Autodesk Inventor part; units mm, degrees
ref_plane "YZ Plane" through (0, 0, 0) normal (1, 0, 0) x (0, 1, 0)
ref_plane "XZ Plane" through (0, 0, 0) normal (0, 1, 0) x (-1, 0, 0)
ref_plane "XY Plane" through (0, 0, 0) normal (0, 0, 1) x (1, 0, 0)
sketch "Sketch1" plane through (0, 0, 0) normal (0, 1, 0) x (-1, 0, 0)
  line L0 (10, -18.5) -> (-10, -18.5)
  line L1 (-10, -18.5) -> (-10, 18.5)
  line L2 (-10, 18.5) -> (10, 18.5)
  line L3 (10, 18.5) -> (10, -18.5)
  point P0 (0, 0)
  dimension "d0" = 20
  dimension "d1" = 37
  dimension "d2" = 18.5
  dimension "d3" = 10
extrude "Plate1" add sketch "Sketch1" along normal blind 1.5
sketch "Sketch2" plane through (-10, 0, -20) normal (0, 0, 1) x (1, 0, 0)
  line L0 (20, 0) -> (0, 0)
  line L1 (0, 0) -> (0, 51.6)
  line L2 (0, 51.6) -> (20, 51.6)
  line L3 (20, 51.6) -> (20, 0)
edge flange "Flange1" height 51.6 angle 90 thickness 1.5 bend radius 0.31 thickness toward (0, 0, 1) relief tear relief width 1.5 relief depth 0.75 edges at (0, 1.5, -18.5) wall of the first edge with corners at (10, 0, -20) (-10, 0, -20) (-10, 51.6, -20) (10, 51.6, -20)
bend "Bend1"
corner "Corner1"
sketch "Sketch3" plane through (10, 0, 20) normal (0, 0, -1) x (-1, 0, 0)
  line L0 (20, 0) -> (0, 0)
  line L1 (0, 0) -> (0, 51.6)
  line L2 (0, 51.6) -> (20, 51.6)
  line L3 (20, 51.6) -> (20, 0)
edge flange "Flange2" height 51.6 angle 90 thickness 1.5 bend radius 0.31 thickness toward (0, 0, -1) relief tear relief width 1.5 relief depth 0.75 edges at (0, 1.5, 18.5) wall of the first edge with corners at (-10, 0, 20) (10, 0, 20) (10, 51.6, 20) (-10, 51.6, 20)
bend "Bend2"
corner "Corner2"
sketch "Sketch4" plane through (-10, 51.6, 20) normal (0, 0, 1) x (1, 0, 0)
  circle A0 centre (10, -10) radius 10
  line L0 (0, 0) -> (20, 0)
  line L1 (0, 0) -> (20, 0)
  line L2 (20, 0) -> (20, -10)
  line L3 (20, -10) -> (0, -10)
  line L4 (0, -10) -> (0, 0)
  line L5 (0, -49.79) -> (0, 0)
  point P0 (10, -51.6)
  point P1 (10, 0)
  dimension "d26" = 20
  dimension "d25" = 10
  dimension "d27" = 10
  dimension "d28" = 10
extrude "Extrusion1" cut sketch "Sketch4" against normal blind 10 contours L4 L0 A0 | A0 L0 L2
sketch "Sketch5" plane through (10, 51.6, -20) normal (0, 0, -1) x (-1, 0, 0)
  arc A0 (20, -10) -> (0, -10) centre (10, -10) ccw
  point P0 (10, -51.6)
hole "Hole1" at (0, 41.6, -20) direction (0, 0, 1) diameter 12.8 depth 1.5
sketch "Sketch6" plane through (10, 51.6, -20) normal (0, 0, -1) x (-1, 0, 0)
  line L0 (0, 0) -> (20, 0)
  circle A0 centre (10, -10) radius 6.4
  line L1 (-4, 0) -> (24, 0)
  line L2 (24, 0) -> (24, -10)
  line L3 (24, -10) -> (-4, -10)
  line L4 (-4, -10) -> (-4, 0)
  line L5 (0, -49.79) -> (0, 0)
  line L6 (0, -49.79) -> (20, -49.79)
  point P0 (10, -51.6)
  dimension "d38" = 28
  dimension "d39" = 10
  dimension "d40" = 4
  dimension "d41" = 49.79
extrude "Extrusion2" cut sketch "Sketch6" against normal blind 10 contours L5 L3 L4 L1 | L0 L1 L2 L3 A0 L5 | A0 L3 picked at (9.2435, -8.0053)
sketch "Sketch7" plane through (-10, 1.81, -18.5) normal (0, 0, 1) x (1, 0, 0)
  circle A0 centre (10, 12.37) radius 0.7835
  circle A1 centre (17, 19.67) radius 0.7835
  line L0 (16.4, 39.79) -> (20, 39.79)
  line L1 (20, 0) -> (20, 39.79)
  line L2 (20, 0) -> (0, 0)
  line L3 (0, 39.79) -> (0, 0)
  line L4 (0, 39.79) -> (3.6, 39.79)
  arc A2 (3.6, 39.79) -> (16.4, 39.79) centre (10, 39.79) ccw
  circle A3 centre (3, 19.67) radius 0.7835
  circle A4 centre (2, 32.89) radius 0.7835
  circle A5 centre (18, 32.89) radius 0.7835
  point P0 (10, -1.81)
hole "Hole2" at (0, 14.18, -18.5) at (-7, 21.48, -18.5) at (-8, 34.7, -18.5) at (8, 34.7, -18.5) at (7, 21.48, -18.5) direction (0, 0, -1) diameter 2.1 depth 1.5
fillet "Fillet1" radius 1 2 edges at (-10, 41.6, -19.25) (10, 41.6, -19.25)
sketch "Sketch8" plane through (-10, 1.81, 20) normal (0, 0, 1) x (1, 0, 0)
  arc A0 (20, 39.79) -> (0, 39.79) centre (10, 39.79) ccw
  point P0 (10, -1.81)
hole "Hole3" at (0, 41.6, 20) direction (0, 0, -1) diameter 3 depth 1.5
sketch "Sketch9" plane through (0, 0, 0) normal (0, -1, 0) x (1, 0, 0)
  line L0 (10.07, -24.6) -> (10.07, 7.5)
  line L1 (10, 20) -> (-10, 20)
  line L2 (10, 18.19) -> (10, -18.19)
  point P0 (0, 0)
  point P1 (8, 9.5)
  point P2 (8, -6.5)
  point P3 (-8, 9.5)
  point P4 (-8, -6.5)
  dimension "d59" = 2
  dimension "d60" = 10.5
  dimension "d63" = 16
  dimension "d66" = 16
hole "Hole4" at (8, 0, 9.5) at (8, 0, -6.5) at (-8, 0, 9.5) at (-8, 0, -6.5) direction (0, 1, 0) diameter 2.1 depth 1.5
equation "\"d36\" = Thickness"
equation "\"d49\" = Thickness"
equation "\"d57\" = Thickness"
equation "\"d74\" = Thickness"
equation "\"d4\" = Thickness"
equation "\"d5\" = BendReliefWidth"
equation "\"d6\" = BendReliefDepth"
equation "\"d7\" = MinimumRemnant"
equation "\"d8\" = TransitionRadius"
equation "\"d11\" = BendRadius"
equation "\"d12\" = CornerReliefSize"
equation "\"d13\" = GapSize"
equation "\"d14\" = JacobiRadiusSize"
equation "\"d15\" = BendReliefWidth"
equation "\"d16\" = BendReliefDepth"
equation "\"d17\" = MinimumRemnant"
equation "\"d18\" = TransitionRadius"
equation "\"d21\" = BendRadius"
equation "\"d22\" = CornerReliefSize"
equation "\"d23\" = GapSize"
equation "\"d24\" = JacobiRadiusSize"
equation "\"BendReliefWidth\" = Thickness"
equation "\"BendReliefDepth\" = 0.5 * Thickness"
equation "\"CornerReliefSize\" = 4 * Thickness"
equation "\"MinimumRemnant\" = 2 * Thickness"
equation "\"TransitionRadius\" = BendRadius"
equation "\"JacobiRadiusSize\" = BendRadius"
equation "\"GapSize\" = Thickness"
properties part number "axis_9_bottom_frame" material "Aluminum 6061-AHC"
Here's how the part is built. I have some questions about the finished solid (model axes, mm). A direction names the side the tool comes from. Round coordinates to 2 decimals unless told otherwise and drop trailing zeros. Loops run counter-clockwise (first coordinate to the right, second up) from the corner with the lowest first, then second, coordinate; pieces in that order, holes last. Notation, with made-up numbers: M 35.25,40 L 43.25,40 A14 ccw 43.25,57 Z; hole C 71,-28.75 d6. An arc over 180 degrees is marked long. Write each question's results on one line, items separated by ' | '. Start each with the question number.
(1) I want a section at A-A (y = 14.18). Please give me the cut outline in (x, z).
(2) If I drill on probe 1 along X at (y, z) = (1.1, -6.5); probe 2 along X at (y, z) = (21.48, -19.1); probe 3 along Z at (x, y) = (-2, 27.5), over which ranges is the centre line in solid material (lowest first)? Write a range as from..to.
(3) I want a section at D-D (y = 5). Please give me the cut outline in (x, z), then the cut area to 3 significant figures.
(4) I want a section at B-B (z = 9.5). Please give me the cut outline in (x, y).
(5) Will these pins go through, and if not, where does the flat tip stop? P1, Ø4, axis at x = 0, y = 41.6, coming from the -Z side; P2, Ø0.8, axis at x = 8, z = -19, coming from the +Y side; P3, Ø6, axis at y = 22, z = -13, coming from the +X side; P4, Ø3.5, axis at x = -8, z = 9.5, coming from the +Y side.
(6) I want a section at C-C (x = 0). Please give me the cut outline in (y, z).
(7) On a 3-axis mill with a long thin cutter (end or side, diameter ignored), from which of +Z, -Z, +X, -X, +Y, -Y can I reach the whole of each face in a straight line? I mean faces 4 (the cylindrical face through (-8.32, 33.7, -19.26)), 5 (the flat face through (8, 41.6, -19)), 6 (the flat face through (0, 1.5, 0)), 7 (the cylindrical face through (-0.1, 35.2, -19.2)). Say none if no direction works.
(8) Thinking about a two-plate mould opening in X: for faces 1 (the flat face through (0, 22, -20)), 2 (the flat face through (10, 1, 0)), 3 (the cylindrical face through (-0.45, 40.17, 19.24)), which applies, pulls with the +X half, pulls with the -X half, needs draft (parallel to the pull), parting line crosses it, or undercut?
Solved:
1) outline: M -10,-20 L -1.05,-20 L -1.05,-18.5 L -10,-18.5 Z; M -10,18.5 L 10,18.5 L 10,20 L -10,20 Z; M 1.05,-20 L 10,-20 L 10,-18.5 L 1.05,-18.5 Z
2) probe 1: x = -10..-9.05, -6.95..6.95, 9.05..10 | probe 2: x = -10..-8.05, -5.95..5.95, 8.05..10 | probe 3: z = -20..-18.5, 18.5..20
3) outline: M -10,-20 L 10,-20 L 10,-18.5 L -10,-18.5 Z; M -10,18.5 L 10,18.5 L 10,20 L -10,20 Z | area: 60.0 mm²
4) outline: M -10,0 L -9.05,0 L -9.05,1.5 L -10,1.5 Z; M -6.95,0 L 6.95,0 L 6.95,1.5 L -6.95,1.5 Z; M 9.05,0 L 10,0 L 10,1.5 L 9.05,1.5 Z
5) P1: stops at z = 18.5 | P2: stops at y = 41.6 | P3: passes through | P4: stops at y = 1.5
6) outline: M 0,-18.19 A1.81 ccw 1.81,-20 L 13.13,-20 L 13.13,-18.5 L 1.81,-18.5 A0.31 cw 1.5,-18.19 L 1.5,18.19 A0.31 cw 1.81,18.5 L 40.1,18.5 L 40.1,20 L 1.81,20 A1.81 ccw 0,18.19 Z; M 15.23,-20 L 35.2,-20 L 35.2,-18.5 L 15.23,-18.5 Z; M 43.1,18.5 L 51.6,18.5 L 51.6,20 L 43.1,20 Z
7) face 4: -Z | face 5: -Z, +X, -X, +Y | face 6: +X, -X, +Y | face 7: -Z, +Y
8) face 1: needs draft | face 2: pulls with the +X half | face 3: undercut
